```python
from build123d import *

# Parameters (mm, degrees)
SKETCH1_R           = 50
BOSS_EXTRUDE1_DEPTH = 60
BOSS_EXTRUDE4_DEPTH = 2
BOSS_EXTRUDE5_DEPTH = 2
BOSS_EXTRUDE6_DEPTH = 2


with BuildPart() as part:
    # Sketch1 → Boss-Extrude1 (new body)
    with BuildSketch(Plane.XY):
        Circle(SKETCH1_R)
    extrude(amount=BOSS_EXTRUDE1_DEPTH)

    # Sketch4 → Boss-Extrude4 (add, symmetric)
    with BuildSketch(Plane(origin=(0, 0, 45), x_dir=(-1, 0, 0), z_dir=(0, 0, -1))):
        with BuildLine():
            Line((-17.101007166, 46.984631039), (-34.465824933, 145.465406341))
            ThreePointArc((-34.465824933, 145.465406341), (0, 155.249311955), (34.465824933, 145.465406341))
            Line((34.465824933, 145.465406341), (17.101007166, 46.984631039))
            ThreePointArc((17.101007166, 46.984631039), (0, 50), (-17.101007166, 46.984631039))
        make_face()
    extrude(amount=BOSS_EXTRUDE4_DEPTH, both=True)

    # Sketch5 → Boss-Extrude5 (add, symmetric)
    with BuildSketch(Plane(origin=(0, 0, 30), x_dir=(-1, 0, 0), z_dir=(0, 0, -1))):
        with BuildLine():
            Line((-32.139380484, -38.302222156), (-108.743824796, -102.580983125))
            ThreePointArc((-108.743824796, -102.580983125), (-134.449848073, -77.624655977), (-143.209649729, -42.884423216))
            Line((-143.209649729, -42.884423216), (-49.240387651, -8.682408883))
            ThreePointArc((-49.240387651, -8.682408883), (-43.301270189, -25), (-32.139380484, -38.302222156))
        make_face()
    extrude(amount=BOSS_EXTRUDE5_DEPTH, both=True)

    # Sketch6 → Boss-Extrude6 (add, symmetric)
    with BuildSketch(Plane(origin=(0, 0, 15), x_dir=(-1, 0, 0), z_dir=(0, 0, -1))):
        with BuildLine():
            Line((49.240387651, -8.682408883), (143.209649729, -42.884423216))
            ThreePointArc((143.209649729, -42.884423216), (134.449848073, -77.624655977), (108.743824796, -102.580983125))
            Line((108.743824796, -102.580983125), (32.139380484, -38.302222156))
            ThreePointArc((32.139380484, -38.302222156), (43.301270189, -25), (49.240387651, -8.682408883))
        make_face()
    extrude(amount=BOSS_EXTRUDE6_DEPTH, both=True)


solid = part.part
```
Input: part model. Units: mm. Frame: model coordinates. A direction names the side the tool comes from. Coordinates: 2 decimals unless noted, no trailing zeros. Loops run counter-clockwise (first coordinate to the right, second up) from the corner with the lowest first, then second, coordinate; pieces in that order, holes last. Notation, with made-up numbers: (2, -37) -> (60, -37) arc R10 cw to (60, -29) -> close; hole circle Ø1 at (24, 7). An arc over 180 degrees is marked (long way). Use a Markdown table: item, result.
1) Cut plane B-B (y = 0). Return the cut outline in (x, z), then the cut area to 3 significant figures.
Results found:
| item | result |
|---|---|
| outline | (-50, 0) -> (50, 0) -> (50, 60) -> (-50, 60) -> close |
| area | 6,000 mm2 |
2) Cut plane D-D (x = -39). Return the cut outline in (y, z).
Results found:
| item | result |
|---|---|
| outline | (-44.06, 13) -> (-31.29, 13) -> (-31.29, 0) -> (31.29, 0) -> (31.29, 60) -> (-31.29, 60) -> (-31.29, 17) -> (-44.06, 17) -> close |
3) Access query for faces 4 (the flat face through (-25.905, 96.914, 44.972)), 5 (the flat face through (69.905, -69.992, 29.972)), 6 (the flat face through (87, -55, 28)), 7 (the cylindrical face through (-6.509, 49.575, 29.58)). Directions: +Z, -Z, +X, -X, +Y, -Y. A direction counts if a zero-diameter tool reaches every point of the face in a straight line with its end or side. Return the directions, or none.
Results found:
| item | result |
|---|---|
| face 4 | +Z, -Z, -X |
| face 5 | +Z, -Z, -Y |
| face 6 | -Z, +X, -Y |
| face 7 | none |
4) Contact query for flat-ended pins moving along their axis: pin 1 (12 mm diameter, centred on x = -46.5, z = 43.5, fed in from -Y); pin 2 (1.5 mm diameter, centred on x = 114, y = -76, fed in from -Z); pin 3 (1 mm diameter, centred on x = 109.5, z = 30.5, fed in from -Y). Output: stop coordinate, or through.
Results found:
| item | result |
|---|---|
| pin 1 | stops at y = -29.32 |
| pin 2 | stops at z = 28 |
| pin 3 | stops at y = -102.44 |
5) Material intervals for line 1 along Z through (x, y) = (-76, -53.5); line 2 along Z through (x, y) = (-3.5, 110); line 3 along Y through (x, z) = (27.5, 51), sorted ascending. Write a range as from..to.
Results found:
| item | result |
|---|---|
| line 1 | z = 13..17 |
| line 2 | z = 43..47 |
| line 3 | y = -41.76..41.76 |
6) Cut plane A-A (x = 0). Return the cut outline in (y, z).
Results found:
| item | result |
|---|---|
| outline | (-50, 0) -> (50, 0) -> (50, 43) -> (155.25, 43) -> (155.25, 47) -> (50, 47) -> (50, 60) -> (-50, 60) -> close |
7) Pull-direction query (Y, two-part tool) for faces 1 (the flat face through (-88, -55, 13)), 2 (the cylindrical face through (0.508, 155.247, 44.972)), 3 (the flat face through (25.662, 95.536, 44.972)); classes: released by +Y, released by -Y, zero draft, split by the parting line, or undercut.
Results found:
| item | result |
|---|---|
| face 1 | zero draft |
| face 2 | released by +Y |
| face 3 | undercut |
8) Cut plane C-C (z = 5). Return the cut outline in (x, y), then the cut area to 3 significant figures.
Results found:
| item | result |
|---|---|
| outline | circle Ø100 at (0, 0) |
| area | 7,850 mm2 |
